from build123d import *

# Parameters (mm, degrees)
F0_W     = 12.7
F0_H     = 6.35
F0_H_2   = 25.4
F0_W_2   = 76.2
F2_R     = 6.35
F3_DEPTH = 101.6


with BuildPart() as f1:
    # F0 (on Top) → F1 (revolve)
    with BuildSketch(Plane.XY):
        with Locations((6.35, -22.225)):
            Rectangle(F0_W, F0_H)
        with Locations((6.35, -38.1)):
            Rectangle(F0_W, F0_H_2)
        with Locations((50.8, -22.225)):
            Rectangle(F0_W_2, F0_H)
        with Locations((95.25, -22.225)):
            Rectangle(F0_W, F0_H)
        with Locations((95.25, -38.1)):
            Rectangle(F0_W, F0_H_2)
    revolve(axis=Axis((50.8, 0, 0), (1, 0, 0)))

    # F2 (on face) → F3 (cut, through all)
    with BuildSketch(Plane(origin=(0, 0, 0), x_dir=(0, -1, 0), z_dir=(-1, 0, 0))):
        with Locations((-28.575, 28.575)):
            Circle(F2_R)
        with Locations((28.575, 28.575)):
            Circle(F2_R)
        with Locations((-28.575, -28.575)):
            Circle(F2_R)
        with Locations((28.575, -28.575)):
            Circle(F2_R)
    extrude(amount=-F3_DEPTH, mode=Mode.SUBTRACT)


solid = f1.part
Geometry check sheet. Reference: the model listing, model coordinates, mm. A direction names the side the tool comes from. Round coordinates to 2 decimals unless told otherwise and drop trailing zeros. Loops run counter-clockwise (first coordinate to the right, second up) from the corner with the lowest first, then second, coordinate; pieces in that order, holes last.
Item 1: Cross-section at C-C on z = 31.5. Record the boundary of the cut face in (x, y), then the cut area to 3 significant figures.
Item 2: Mould release check, pull along Y, two halves, no side actions. Record for faces 1 (the cylindrical face through (6.26, 22.71, 26.14)), 2 (the flat face through (12.7, -10.6, -23.3)), 3 (the cylindrical face through (95.339, 11.012, 49.592)): pulls with the +Y half, pulls with the -Y half, needs draft (parallel to the pull), parting line crosses it, or undercut.
Item 3: Gauge pin test, flat ends, axial feed: pin 1 (6 mm diameter, centred on x = 28.5, y = 1, fed in from +Z); pin 2 (1.5 mm diameter, centred on x = 64.5, z = 17, fed in from -Y); pin 3 (1 mm diameter, centred on x = 28.5, y = 16, fed in from -Z). Record the tip position at first contact, or that the pin passes through.
Item 4: Thickness scan on line 1 (X direction, y = 5.5, z = 26); line 2 (Z direction, x = 9, y = -1); line 3 (Z direction, x = 91, y = 25). Record the ranges inside material, lowest first.
Item 5: Cross-section at A-A on y = 0. Record the boundary of the cut face in (x, z), then the cut area to 3 significant figures.
Item 6: Cross-section at D-D on y = -29. Record the boundary of the cut face in (x, z).
Item 7: Access from +Z, -Z, +X, -X, +Y, -Y to the whole of each face (thin tool, end or side, straight path). Record for faces 4 (the flat face through (88.9, -10.6, -23.3)), 5 (the cylindrical face through (95.161, 22.518, -26.668)).
Answer sheet:
1. outline: (0, -39.85) - (12.7, -39.85) - (12.7, -34.21) - (0, -34.21) - close; (0, -22.94) - (12.7, -22.94) - (12.7, 22.94) - (0, 22.94) - close; (0, 34.21) - (12.7, 34.21) - (12.7, 39.85) - (0, 39.85) - close; (88.9, -39.85) - (101.6, -39.85) - (101.6, -34.21) - (88.9, -34.21) - close; (88.9, -22.94) - (101.6, -22.94) - (101.6, 22.94) - (88.9, 22.94) - close; (88.9, 34.21) - (101.6, 34.21) - (101.6, 39.85) - (88.9, 39.85) - close
1. area: 1,450 mm2
2. face 1: undercut
2. face 2: needs draft
2. face 3: parting line crosses it
3. pin 1: stops at z = 25.4
3. pin 2: stops at y = -19.52
3. pin 3: stops at z = -20.12
4. line 1: x = 0 to 12.7, 88.9 to 101.6
4. line 2: z = -50.79 to -19.02, 19.02 to 50.79
4. line 3: z = -44.22 to -33.82, -23.33 to 23.33, 33.82 to 44.22
5. outline: (0, -50.8) - (12.7, -50.8) - (12.7, -25.4) - (88.9, -25.4) - (88.9, -50.8) - (101.6, -50.8) - (101.6, -19.05) - (0, -19.05) - close; (0, 19.05) - (101.6, 19.05) - (101.6, 50.8) - (88.9, 50.8) - (88.9, 25.4) - (12.7, 25.4) - (12.7, 50.8) - (0, 50.8) - close
5. area: 2,580 mm2
6. outline: (0, -41.71) - (12.7, -41.71) - (12.7, -34.91) - (0, -34.91) - close; (0, -22.24) - (12.7, -22.24) - (12.7, 22.24) - (0, 22.24) - close; (0, 34.91) - (12.7, 34.91) - (12.7, 41.71) - (0, 41.71) - close; (88.9, -41.71) - (101.6, -41.71) - (101.6, -34.91) - (88.9, -34.91) - close; (88.9, -22.24) - (101.6, -22.24) - (101.6, 22.24) - (88.9, 22.24) - close; (88.9, 34.91) - (101.6, 34.91) - (101.6, 41.71) - (88.9, 41.71) - close
7. face 4: none
7. face 5: +X, -X
